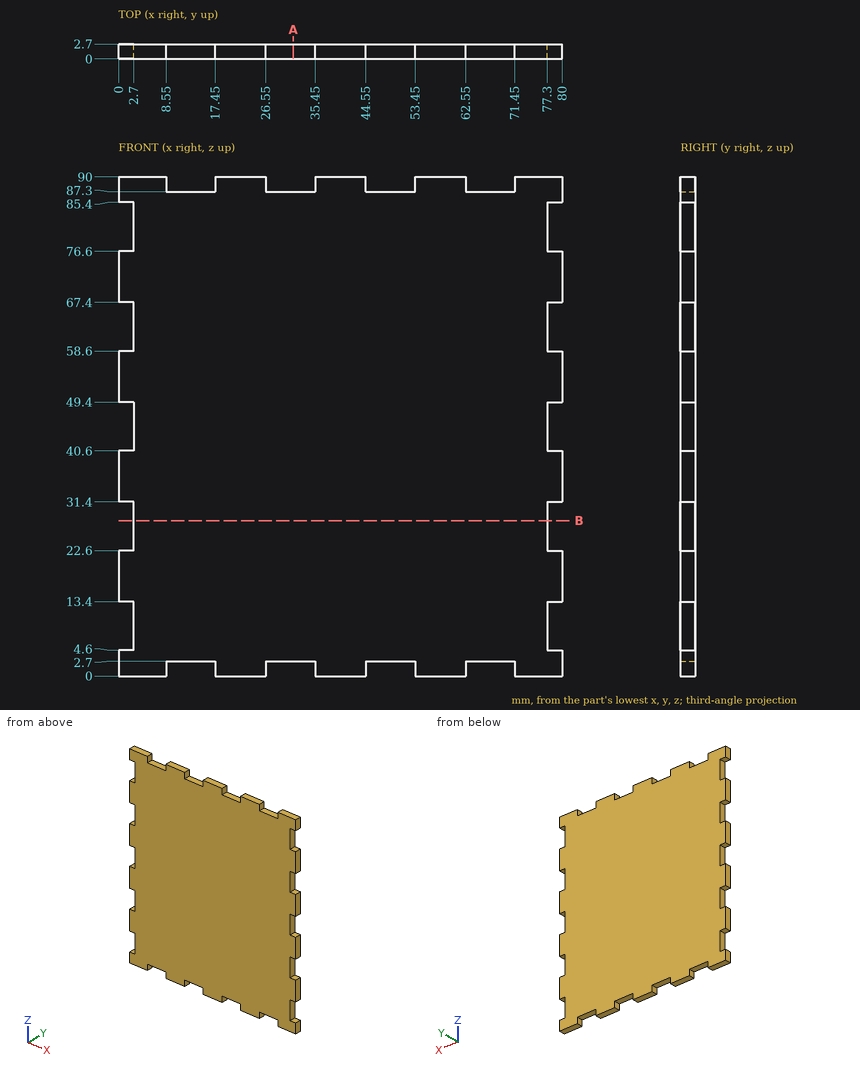
For this review, use the dimensioned drawing (mm, ordinates from the lowest corner) and the shaded views. Give positions to 0.01 mm unless a question says otherwise; leave off trailing zeros. Order: outer loops, then holes, each group sorted by start corner. A loop starts at its lowest first (then second) coordinate and runs counter-clockwise, first axis right, second up. Notation, with made-up numbers: (-34, 4) - (24, 4) arc R27 ccw to (24, 29) - close; hole circle Ø7 at (-26.75, 45.5). An arc over 180 degrees is marked (long way). Use CSV: the item, a comma, the result in double quotes. Start each with the question number.
Q1. We need section B-B, the plane z = 28. Write out the cut boundary in (x, y), and give its area (3 significant figures).
Q2. We need section A-A, the plane x = 31.5. Write out the cut boundary in (y, z), and give its area (3 significant figures).
Q3. To check wall thickness, follow line 1 along X through (y, z) = (0.75, 9); line 2 along Z through (x, y) = (70, 0.6). State the ranges of each line that lie inside material, in increasing order. Write a range as [from, to].
Q4. Clearance check with flat-ended pins moving along their axes: pin 1 Ø1 at (y, z) = (2.5, 60.5) entering from +X; pin 2 Ø10 at (x, z) = (41, 15.5) entering from -Y; pin 3 Ø0.8 at (x, y) = (32.5, 1) entering from +Z; pin 4 Ø1.4 at (x, y) = (13.5, 1.5) entering from -Z. State where each tip first meets the part, or that it passes through.
Outcome:
1,outline,"(2.7, 0) - (77.3, 0) - (77.3, 2.7) - (2.7, 2.7) - close"
1,area,"201 mm^2"
2,outline,"(0, 2.7) - (2.7, 2.7) - (2.7, 87.3) - (0, 87.3) - close"
2,area,"228 mm^2"
3,line 1,"x = [2.7, 77.3]"
3,line 2,"z = [2.7, 87.3]"
4,pin 1,"stops at x = 77.3"
4,pin 2,"stops at y = 0"
4,pin 3,"stops at z = 87.3"
4,pin 4,"stops at z = 2.7"
